Can you work these out from the model? Positions are in its coordinate system, mm. A direction names the side the tool comes from. Give positions to 0.01 mm unless a question says otherwise; leave off trailing zeros. Write each loop counter-clockwise with the first axis right and the second up, starting at its lowest first coordinate (ties: lowest second). Pieces come first, ordered by that corner, then holes. Notation, with made-up numbers: (34, 71) -> (93, 71) arc R18 ccw to (93, 79) -> close; hole circle Ø10 at (19, -23.75). An arc over 180 degrees is marked (long way). Answer as CSV lines item,"result". Start each with the question number.
1. If we section it at A-A on x = 25.5: Write out the boundary of the cut face in (y, z).
2. I'm going to push flat-ended pins straight in: P1, Ø8, axis at y = -3.5, z = 4, coming from the -X side; P2, Ø1.5, axis at x = 14.5, y = -10, coming from the +Z side; P3, Ø12, axis at x = -32, y = 7.5, coming from the +Z side; P4, Ø8, axis at y = 8, z = -11.5, coming from the -X side. Where does each tip first touch, or does it pass through?
3. If we section it at B-B on z = 0: Write out the boundary of the cut face in (x, y), plus the area to 3 significant figures.
4. If we section it at D-D on x = -16.5: Write out the boundary of the cut face in (y, z).
5. If we section it at C-C on y = 0: Write out the boundary of the cut face in (x, z), plus the area to 3 significant figures.
6. On a 3-axis mill with a long thin cutter (end or side, diameter ignored), from which of +Z, -Z, +X, -X, +Y, -Y can I reach the whole of each face in a straight line? I mean faces 1 (the face through (-38, 2.5, 0)), 2 (the face through (0, 0, 14)), 3 (the face through (17, 0, -13)), 4 (the face through (4, 0, 14)), 5 (the face through (16.82, -12.57, -12.55)). Say none if no direction works.
7. I need wall thicknesses on line 1 (Y direction, x = 0.7, z = 0); line 2 (Z direction, x = 12.5, y = -8.25). Which ranges of each line are inside material? Lowest first, please. Write a range as [from, to].
```python
from build123d import *

# Parameters (mm, degrees)
SKETCH_1_W          = 30
SKETCH_1_H          = 30
EXTRUDE_1_DEPTH     = 30
SKETCH_2_R          = 12
EXTRUDE_2_DEPTH     = 25
SKETCH_3_R          = 13
SKETCH_3_R_2        = 12
CUT_EXTRUDE_1_DEPTH = 1
FILLET_1_R          = 2
FILLET_2_R          = 1
SKETCH_5_W          = 30
SKETCH_5_H          = 30
SKETCH_5_W_2        = 26
SKETCH_5_H_2        = 26
CUT_EXTRUDE_2_DEPTH = 26
FILLET_3_R          = 1.5
SKETCH_4_R          = 3
EXTRUDE_3_DEPTH     = 15
SKETCH_6_W          = 3.31662479
SKETCH_6_H          = 0.5
CUT_EXTRUDE_3_DEPTH = 5


with BuildPart() as part:
    # 草图1 → 凸台-拉伸1 (new body)
    with BuildSketch(Plane(origin=(0, 0, 0), x_dir=(0, 0, -1), z_dir=(1, 0, 0))):
        Rectangle(SKETCH_1_W, SKETCH_1_H)
    extrude(amount=EXTRUDE_1_DEPTH)

    # 草图2 → 凸台-拉伸2 (add)
    with BuildSketch(Plane.ZY):
        Circle(SKETCH_2_R)
    extrude(amount=EXTRUDE_2_DEPTH)

    # 草图3 → 切除-拉伸1 (cut)
    with BuildSketch(Plane.ZY):
        Circle(SKETCH_3_R)
        Circle(SKETCH_3_R_2, mode=Mode.SUBTRACT)
    extrude(amount=-CUT_EXTRUDE_1_DEPTH, mode=Mode.SUBTRACT)

    # 圆角1
    fillet_1_edges = [part.edges().sort_by_distance(p)[0] for p in [
        (15, 15, 15),
        (15, 15, -15),
        (15, -15, -15),
        (15, -15, 15),
    ]]
    fillet(fillet_1_edges, radius=FILLET_1_R)

    # 圆角2
    fillet_2_edges = [part.edges().sort_by_distance(p)[0] for p in [
        (-25, 0, -12),
    ]]
    fillet(fillet_2_edges, radius=FILLET_2_R)

    # 草图5 → 切除-拉伸2 (cut)
    with BuildSketch(Plane(origin=(30, 0, 0), x_dir=(0, 0, -1), z_dir=(1, 0, 0))):
        Rectangle(SKETCH_5_W, SKETCH_5_H)
        Rectangle(SKETCH_5_W_2, SKETCH_5_H_2, mode=Mode.SUBTRACT)
    extrude(amount=-CUT_EXTRUDE_2_DEPTH, mode=Mode.SUBTRACT)

    # 圆角3
    fillet_3_edges = [part.edges().sort_by_distance(p)[0] for p in [
        (17, 13, 13),
        (17, 13, -13),
        (17, -13, -13),
        (17, -13, 13),
    ]]
    fillet(fillet_3_edges, radius=FILLET_3_R)

    # 草图4 → 凸台-拉伸3 (add)
    with BuildSketch(Plane.ZY.offset(25)):
        Circle(SKETCH_4_R)
    extrude(amount=EXTRUDE_3_DEPTH)

    # 草图6 → 切除-拉伸3 (cut)
    with BuildSketch(Plane.ZY.offset(40)):
        with Locations((0, 2.75)):
            Rectangle(SKETCH_6_W, SKETCH_6_H)
    extrude(amount=-CUT_EXTRUDE_3_DEPTH, mode=Mode.SUBTRACT)


solid = part.part
```
Computed values:
1,outline,"(-13, -11.5) arc R1.5 ccw to (-11.5, -13) -> (11.5, -13) arc R1.5 ccw to (13, -11.5) -> (13, 11.5) arc R1.5 ccw to (11.5, 13) -> (-11.5, 13) arc R1.5 ccw to (-13, 11.5) -> close"
2,P1,"stops at x = -40"
2,P2,"stops at z = 13"
2,P3,"stops at z = 2.6"
2,P4,"stops at x = -25"
3,outline,"(-40, -3) -> (-25, -3) -> (-25, -11) arc R1 ccw to (-24, -12) -> (1, -12) -> (1, -13) -> (0, -13) -> (0, -15) -> (4, -15) -> (4, -13) -> (30, -13) -> (30, 13) -> (4, 13) -> (4, 15) -> (0, 15) -> (0, 13) -> (1, 13) -> (1, 12) -> (-24, 12) arc R1 ccw to (-25, 11) -> (-25, 3) -> (-35, 3) -> (-35, 2.5) -> (-40, 2.5) -> close"
3,area,"1,480 mm2"
4,outline,"circle Ø24 at (0, 0)"
5,outline,"(-40, -3) -> (-25, -3) -> (-25, -11) arc R1 ccw to (-24, -12) -> (1, -12) -> (1, -13) -> (0, -13) -> (0, -15) -> (4, -15) -> (4, -13) -> (30, -13) -> (30, 13) -> (4, 13) -> (4, 15) -> (0, 15) -> (0, 13) -> (1, 13) -> (1, 12) -> (-24, 12) arc R1 ccw to (-25, 11) -> (-25, 3) -> (-40, 3) -> close"
5,area,"1,480 mm2"
6,face 1,"+Z, -Z, -X, +Y"
6,face 2,"-X"
6,face 3,"-Z, +X, +Y, -Y"
6,face 4,"+X"
6,face 5,"-Z, +X, -Y"
7,line 1,"y = [-15, -13], [-12, 12], [13, 15]"
7,line 2,"z = [-13, 13]"
